```python
from build123d import *

# Parameters (mm, degrees)
F0_W     = 159.44358
F0_H     = 118.819759
F1_DEPTH = 63.5
F2_W     = 44.598654
F2_H     = 64.595787
F3_DEPTH = 66.802
F5_DEPTH = 64.595786
F6_W     = 126.061455
F6_H     = 6.612033
F7_DEPTH = 70.866


with BuildPart() as f1:
    # F0 (on Front) → F1 (new body)
    with BuildSketch(Plane.XZ):
        with Locations((13.00003, -12.35427)):
            Rectangle(F0_W, F0_H)
    extrude(amount=F1_DEPTH)

    # F2 (on face) → F3 (cut)
    with BuildSketch(Plane.XZ.offset(63.5)):
        with Locations((70.422493, 14.757716)):
            Rectangle(F2_W, F2_H)
    extrude(amount=-F3_DEPTH, mode=Mode.SUBTRACT)

    # F4 (on face) → F5 (cut, through all)
    with BuildSketch(Plane.XY.offset(47.05561)):
        Polygon((48.123166, -63.5), (48.123166, 0), (6.32387, -63.5), align=None)
    extrude(amount=-F5_DEPTH, mode=Mode.SUBTRACT)

    # F6 (on face) → F7 (cut)
    with BuildSketch(Plane.XZ.offset(63.5)):
        with Locations((-3.691033, 43.749593)):
            Rectangle(F6_W, F6_H)
    extrude(amount=-F7_DEPTH, mode=Mode.SUBTRACT)


solid = f1.part
```
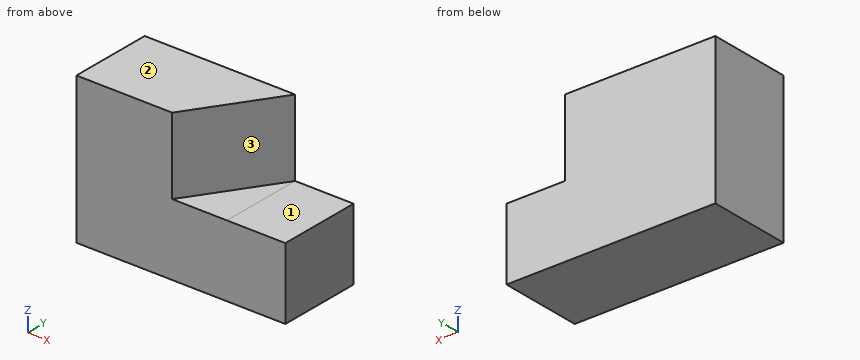
Geometry check sheet. Reference: the model listing, model coordinates, mm. Face numbers are marked on the shaded views. A direction names the side the tool comes from. Round coordinates to 2 decimals unless told otherwise and drop trailing zeros. Order: outer loops, then holes, each group sorted by start corner. A loop starts at its lowest first (then second) coordinate and runs counter-clockwise, first axis right, second up. Notation, with made-up numbers: (3, -3) -> (40, -3) arc R22 cw to (40, 9) -> close; hole circle Ø4 at (-18, -1). An arc over 180 degrees is marked (long way). Return JSON: item names as keys, results as strings. Group by question number.
Q1. Material ranges on probe 1 along Z at (x, y) = (62, -40.5); probe 2 along X at (y, z) = (-57, 10); probe 3 along X at (y, z) = (-59, 25.5), recorded low to high. Write a range as from..to.
Q2. Tool access check on the marked faces 1, 2 and 3. Record the directions out of +Z, -Z, +X, -X, +Y, -Y that give a thin tool (end or side, any length) a straight path to the whole face; none if there is none.
Q3. Section check C-C, the plane z = -1. Record the boundary of the cut face in (x, y).
Q4. Section check B-B, the plane x = 14. Record the boundary of the cut face in (y, z).
Q5. Gauge pin test, flat ends, axial feed: pin 1 (12.5 mm diameter, centred on x = 36, y = -39, fed in from +Z); pin 2 (10 mm diameter, centred on y = -31.5, z = -11.5, fed in from +X); pin 3 (10 mm diameter, centred on y = -25.5, z = 29, fed in from +X). Record the tip position at first contact, or that the pin passes through.
Numbers:
{
 "1": {"probe 1": "-71.76..-17.54", "probe 2": "-66.72..10.6", "probe 3": "-66.72..9.29"},
 "2": {"face 1": "+Z, +X, +Y, -Y", "face 2": "+Z, +X, -X, +Y, -Y", "face 3": "+Z, +X, -Y"},
 "3": {"outline": "(-66.72, -63.5) -> (6.32, -63.5) -> (48.12, 0) -> (-66.72, 0) -> close"},
 "4": {"outline": "(-63.5, -71.76) -> (0, -71.76) -> (0, 40.44) -> (-51.84, 40.44) -> (-51.84, -17.54) -> (-63.5, -17.54) -> close"},
 "5": {"pin 1": "z = -17.54", "pin 2": "x = 30.68", "pin 3": "x = 34.63"}
}
